from build123d import *

# Parameters (mm, degrees)
SKETCH1_W               = 12.7
SKETCH1_H               = 12.7
BOSS_EXTRUDE1_DEPTH     = 12.7
SKETCH3_W               = 3.81
SKETCH3_H               = 8.89
CUT_EXTRUDE1_DEPTH      = 93.361399405
SKETCH4_W               = 4.445
SKETCH4_H               = 9.525
CUT_EXTRUDE2_DEPTH      = 12.7
SKETCH5_R               = 3.175
CUT_EXTRUDE3_DEPTH      = 12.7
BOSS_EXTRUDE3_DEPTH     = 12.7
BOSS_EXTRUDE2_START     = -6.35
BOSS_EXTRUDE2_OUTLINE_R = 5.08
BOSS_EXTRUDE2_DEPTH     = 6.35


# Read off the part's stored shape, not the designer's step: Boss-Extrude2
with BuildPart() as part:
    # Sketch1 → Boss-Extrude1 (new body)
    with BuildSketch(Plane.XY):
        with Locations((6.35, 6.35)):
            Rectangle(SKETCH1_W, SKETCH1_H)
        Polygon((12.7, 12.7), (12.7, 0), (12.7, -8.89), (101.6, -8.89), (101.6, -6.35), (15.24, -6.35), (15.24, 19.05), (101.6, 19.05), (101.6, 21.59), (12.7, 21.59), align=None)
    extrude(amount=BOSS_EXTRUDE1_DEPTH)

    # Sketch3 → Cut-Extrude1 (cut, through all)
    with BuildSketch(Plane.ZY.offset(-12.7)):
        with Locations((1.905, 17.145)):
            Rectangle(SKETCH3_W, SKETCH3_H)
        with Locations((10.795, 17.145)):
            Rectangle(SKETCH3_W, SKETCH3_H)
        with Locations((10.795, -4.445)):
            Rectangle(SKETCH3_W, SKETCH3_H)
        with Locations((1.905, -4.445)):
            Rectangle(SKETCH3_W, SKETCH3_H)
    extrude(amount=-CUT_EXTRUDE1_DEPTH, mode=Mode.SUBTRACT)

    # Sketch4 → Cut-Extrude2 (cut)
    with BuildSketch(Plane(origin=(15.24, 0, 0), x_dir=(0, 0, -1), z_dir=(1, 0, 0))):
        with Locations((-6.35, 6.35)):
            Rectangle(SKETCH4_W, SKETCH4_H)
    extrude(amount=-CUT_EXTRUDE2_DEPTH, mode=Mode.SUBTRACT)

    # Sketch5 → Cut-Extrude3 (cut)
    with BuildSketch(Plane.XY.offset(12.7)):
        with Locations((10.4775, 6.35)):
            Circle(SKETCH5_R)
    extrude(amount=-CUT_EXTRUDE3_DEPTH, mode=Mode.SUBTRACT)

    # Sketch7 → Boss-Extrude3 (add)
    with BuildSketch(Plane(origin=(0, 12.7, 0), x_dir=(1, 0, 0), z_dir=(0, 1, 0))):
        Polygon((0, -2.683825791), (-3.175, -8.183087105), (0, -10.016174209), align=None)
    extrude(amount=-BOSS_EXTRUDE3_DEPTH)

    # Boss-Extrude2 outline → Boss-Extrude2 (add)
    with BuildSketch(Plane(origin=(0.622783942, 0, 10.375738686), x_dir=(0.8660254037844416, 0, 0.499999999999995), z_dir=(-0.49999999999999495, 0, 0.8660254037844415)).offset(BOSS_EXTRUDE2_START)):
        with BuildLine():
            Line((-0.719128953, 12.7), (-14.545303163, 12.7))
            ThreePointArc((-14.545303163, 12.7), (-20.895303163, 6.35), (-14.545303163, 0))
            Line((-14.545303163, 0), (-0.719128953, 0))
            Line((-0.719128953, 0), (-0.719128953, 12.7))
        make_face()
        with Locations((-14.545303163, 6.35)):
            Circle(BOSS_EXTRUDE2_OUTLINE_R, mode=Mode.SUBTRACT)
    extrude(amount=BOSS_EXTRUDE2_DEPTH)


solid = part.part
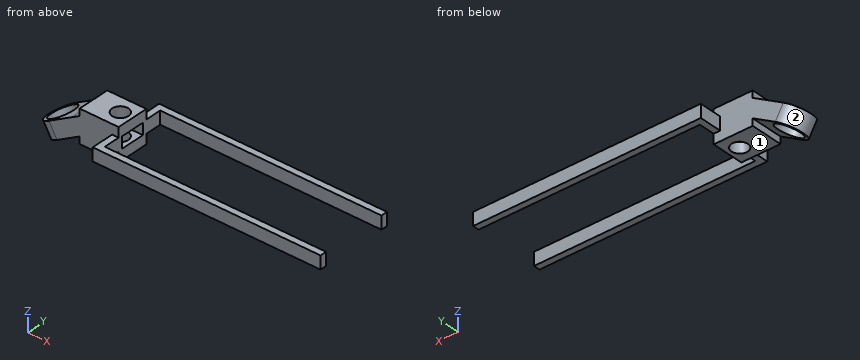
For this review, take the finished solid that the model builds, in its own axes (mm). Face numbers are marked on the shaded views. A direction names the side the tool comes from. Coordinates: 2 decimals unless noted, no trailing zeros. Loops run counter-clockwise (first coordinate to the right, second up) from the corner with the lowest first, then second, coordinate; pieces in that order, holes last. Notation, with made-up numbers: (78, -28) - (118, -28) arc R20 cw to (118, 5) - close; hole circle Ø11 at (9, 23). An arc over 180 degrees is marked (long way). Use a Markdown table: item, result. Add a question column.
Item 1: Insertion check: pin 1 Ø10 at (x, y) = (72.5, 17) entering from +Z; pin 2 Ø2.5 at (y, z) = (19.5, 6.5) entering from -X; pin 3 Ø6 at (x, z) = (-5.5, 1.5) entering from +Y; pin 4 Ø7.5 at (x, y) = (10.48, 6.35) entering from +Z. Each pin has a flat end and moves straight along its axis. Give the tip position at first contact, or say it passes through.
Item 2: For line 1 (Y direction, x = 62.5, z = 5.75); line 2 (X direction, y = 6.5, z = 1.75); line 3 (Z direction, x = 14.5, y = 20.5), list the stretches that pass through material, from the lowest coordinate up.
Item 3: We need section B-B (y = 6.35). Give the number of separate pieces and of enclosed holes in the cut face, and give its area (3 significant figures).
Item 4: We need section C-C (x = 32.5). Give the boundary of the cut face in (y, z), and give its area (3 significant figures).
Item 5: Tool access review of the marked faces 1 and 2: name each direction out of +Z, -Z, +X, -X, +Y, -Y from which nothing blocks a thin tool from reaching the whole face with its end or side.
Item 6: We need section A-A (x = 9). Give the boundary of the cut face in (y, z).
Results list:
| question | item | result |
|---|---|---|
| 1 | pin 1 | stops at z = 8.89 |
| 1 | pin 2 | stops at x = 12.7 |
| 1 | pin 3 | stops at y = 12.7 |
| 1 | pin 4 | stops at z = 12.7 |
| 2 | line 1 | y = -8.89 to -6.35, 19.05 to 21.59 |
| 2 | line 2 | x = -5.33 to -1.62, 0 to 7.31, 13.65 to 15.24 |
| 2 | line 3 | z = 3.81 to 8.89 |
| 3 | separate pieces | 4 |
| 3 | enclosed holes | 0 |
| 3 | area | 137 mm^2 |
| 4 | outline | (-8.89, 3.81) - (-6.35, 3.81) - (-6.35, 8.89) - (-8.89, 8.89) - close; (19.05, 3.81) - (21.59, 3.81) - (21.59, 8.89) - (19.05, 8.89) - close |
| 4 | area | 25.8 mm^2 |
| 5 | face 1 | -Z, +X, +Y, -Y |
| 5 | face 2 | -Z, -X |
| 6 | outline | (0, 0) - (3.54, 0) - (3.54, 4.13) - (1.59, 4.13) - (1.59, 8.57) - (3.54, 8.57) - (3.54, 12.7) - (0, 12.7) - close; (9.16, 0) - (12.7, 0) - (12.7, 12.7) - (9.16, 12.7) - (9.16, 8.57) - (11.11, 8.57) - (11.11, 4.13) - (9.16, 4.13) - close |
